Geometry: final body of the model. Coordinates: model frame, mm. A direction names the side the tool comes from. Round coordinates to 2 decimals unless told otherwise and drop trailing zeros. Loops run counter-clockwise (first coordinate to the right, second up) from the corner with the lowest first, then second, coordinate; pieces in that order, holes last. Notation, with made-up numbers: (82.25, 76.5) - (126.25, 76.5) arc R13 ccw to (126.25, 94.5) - close; hole circle Ø1 at (-40, 5). An arc over 180 degrees is marked (long way). Return JSON: item names as keys, results as strings. Group by question number.
1. First-contact query: pin 1 Ø1.5 at (x, z) = (27.5, 2.5) entering from -Y. Flat tip, straight axial feed; report the tip coordinate or a pass-through.
2. Set-up query: faces 4 (the face through (0, 31.5, 2)), 5 (the face through (24, -8, 2)). Return all of +Z, -Z, +X, -X, +Y, -Y with unobstructed straight access to the full face (end or side cutting, diameter ignored); none if empty.
3. Material intervals for probe 1 along X at (y, z) = (26.5, 1.9); probe 2 along Y at (x, z) = (12.5, 2.9), sorted ascending.
4. Section C-C on z = 1.1. Count the separate pieces of the cut face and the enclosed holes in it, and give its area (3 significant figures).
5. Section A-A on y = 0. Return loops of the section in (x, z).
6. Section B-B on x = -8. Return loops of the section in (y, z), and give its area (3 significant figures).
7. Draft query along Y for faces 1 (the face through (0, -31.5, 2)), 2 (the face through (0, 21, 2)), 3 (the face through (-30.07, 30, 2.54)). Return one class per face: +Y half, -Y half, draft (parallel to the pull), parting line (faces both ways), or undercut.
from build123d import *

# Parameters (mm, degrees)
ESQUISSE1_W        = 63
ESQUISSE1_H        = 63
ESQUISSE1_R        = 2
ESQUISSE1_W_2      = 42
ESQUISSE1_H_2      = 42
ESQUISSE1_W_3      = 5
ESQUISSE1_H_3      = 5
BOSS_EXTRU_1_DEPTH = 5
CONG_1_R           = 5


with BuildPart() as part:
    # Esquisse1 → Boss.-Extru.1 (new body)
    with BuildSketch(Plane.XY):
        Rectangle(ESQUISSE1_W, ESQUISSE1_H)
        with Locations((26.5, 0)):
            Circle(ESQUISSE1_R, mode=Mode.SUBTRACT)
        with Locations(Location((-26.5, 0, 0), (0, 0, 180))):
            Circle(ESQUISSE1_R, mode=Mode.SUBTRACT)
        with Locations(Location((0, 26.5, 0), (0, 0, 90))):
            Circle(ESQUISSE1_R, mode=Mode.SUBTRACT)
        with Locations(Location((0, -26.5, 0), (0, 0, 270))):
            Circle(ESQUISSE1_R, mode=Mode.SUBTRACT)
        Rectangle(ESQUISSE1_W_2, ESQUISSE1_H_2, mode=Mode.SUBTRACT)
        with Locations((26.5, 7.5)):
            Rectangle(ESQUISSE1_W_3, ESQUISSE1_H_3, mode=Mode.SUBTRACT)
        with Locations((26.5, -7.5)):
            Rectangle(ESQUISSE1_W_3, ESQUISSE1_H_3, mode=Mode.SUBTRACT)
        with Locations((-26.5, 7.5)):
            Rectangle(ESQUISSE1_W_3, ESQUISSE1_H_3, mode=Mode.SUBTRACT)
        with Locations((-26.5, -7.5)):
            Rectangle(ESQUISSE1_W_3, ESQUISSE1_H_3, mode=Mode.SUBTRACT)
        with Locations((7.5, 26.5)):
            Rectangle(ESQUISSE1_W_3, ESQUISSE1_H_3, mode=Mode.SUBTRACT)
        with Locations((-7.5, 26.5)):
            Rectangle(ESQUISSE1_W_3, ESQUISSE1_H_3, mode=Mode.SUBTRACT)
        with Locations((7.5, -26.5)):
            Rectangle(ESQUISSE1_W_3, ESQUISSE1_H_3, mode=Mode.SUBTRACT)
        with Locations((-7.5, -26.5)):
            Rectangle(ESQUISSE1_W_3, ESQUISSE1_H_3, mode=Mode.SUBTRACT)
    extrude(amount=BOSS_EXTRU_1_DEPTH)

    # Congé1
    cong_1_edges = [part.edges().sort_by_distance(p)[0] for p in [
        (-31.5, 31.5, 2.5),
        (31.5, 31.5, 2.5),
        (31.5, -31.5, 2.5),
        (-31.5, -31.5, 2.5),
    ]]
    fillet(cong_1_edges, radius=CONG_1_R)


solid = part.part
Taken from the geometry:
{
 "1": {"pin 1": "y = -31.49"},
 "2": {"face 4": "+Z, -Z, +X, -X, +Y", "face 5": "+Z, -Z"},
 "3": {"probe 1": "-31.5 to -10, -5 to -2, 2 to 5, 10 to 31.5", "probe 2": "-31.5 to -21, 21 to 31.5"},
 "4": {"separate pieces": "1", "enclosed holes": "13", "area": "1,930 mm2"},
 "5": {"outline": "(-31.5, 0) - (-28.5, 0) - (-28.5, 5) - (-31.5, 5) - close; (-24.5, 0) - (-21, 0) - (-21, 5) - (-24.5, 5) - close; (21, 0) - (24.5, 0) - (24.5, 5) - (21, 5) - close; (28.5, 0) - (31.5, 0) - (31.5, 5) - (28.5, 5) - close"},
 "6": {"outline": "(-31.5, 0) - (-29, 0) - (-29, 5) - (-31.5, 5) - close; (-24, 0) - (-21, 0) - (-21, 5) - (-24, 5) - close; (21, 0) - (24, 0) - (24, 5) - (21, 5) - close; (29, 0) - (31.5, 0) - (31.5, 5) - (29, 5) - close", "area": "55.0 mm2"},
 "7": {"face 1": "-Y half", "face 2": "undercut", "face 3": "+Y half"}
}
